```python
from build123d import *

# Parameters (mm, degrees)
SKETCH1_W           = 200
SKETCH1_H           = 100
BOSS_EXTRUDE1_DEPTH = 5
SKETCH2_W           = 50
SKETCH2_H           = 54
CUT_EXTRUDE1_DEPTH  = 6
SKETCH3_W           = 50
SKETCH3_H           = 4
BOSS_EXTRUDE2_DEPTH = 45
CUT_EXTRUDE3_DEPTH  = 4
SKETCH19_W          = 200
SKETCH19_H          = 5
BOSS_EXTRUDE3_DEPTH = 25
SKETCH20_W          = 200
SKETCH20_H          = 5
BOSS_EXTRUDE4_DEPTH = 25
SKETCH21_W          = 150
SKETCH21_H          = 5
BOSS_EXTRUDE5_DEPTH = 25
SKETCH22_OUTSIDE_W  = 282
SKETCH22_OUTSIDE_H  = 207
SKETCH22_OUTSIDE_R  = 75
CUT_EXTRUDE6_DEPTH  = 51
SKETCH26_R          = 2
CUT_EXTRUDE7_DEPTH  = 51
CUT_EXTRUDE8_REACH  = 52
SKETCH28_R          = 4.2
CUT_EXTRUDE10_DEPTH = 4


with BuildPart() as part:
    # Sketch1 → Boss-Extrude1 (new body)
    with BuildSketch(Plane(origin=(0, 0, 0), x_dir=(1, 0, 0), z_dir=(0, 1, 0))):
        Rectangle(SKETCH1_W, SKETCH1_H)
    extrude(amount=BOSS_EXTRUDE1_DEPTH)

    # Sketch2 → Cut-Extrude1 (cut, through all)
    with BuildSketch(Plane(origin=(0, 5, 0), x_dir=(1, 0, 0), z_dir=(0, 1, 0))):
        with Locations((30, 0)):
            Rectangle(SKETCH2_W, SKETCH2_H)
    extrude(amount=-CUT_EXTRUDE1_DEPTH, mode=Mode.SUBTRACT)

    # Sketch3 → Boss-Extrude2 (add)
    with BuildSketch(Plane.XZ):
        with Locations((30, -29)):
            Rectangle(SKETCH3_W, SKETCH3_H)
    extrude(amount=BOSS_EXTRUDE2_DEPTH)

    # Sketch4 → Cut-Extrude3 (cut)
    with BuildSketch(Plane.XY.offset(-27)):
        with BuildLine():
            ThreePointArc((14, 3.960327286), (11.85, 6.110327286), (9.7, 3.960327286))
            Line((9.7, 3.960327286), (9.7, -6.197738793))
            Line((9.7, -6.197738793), (14, -6.197264156))
            Line((14, -6.197264156), (14, 3.960327286))
        make_face()
        with BuildLine():
            Line((41.7, 3.960327286), (41.7, -31.94922721))
            ThreePointArc((41.7, -31.94922721), (43.85, -34.09922721), (46, -31.94922721))
            Line((46, -31.94922721), (46, 3.960327286))
            ThreePointArc((46, 3.960327286), (43.85, 6.110327286), (41.7, 3.960327286))
        make_face()
    extrude(amount=-CUT_EXTRUDE3_DEPTH, mode=Mode.SUBTRACT)

    # Sketch19 → Boss-Extrude3 (add)
    with BuildSketch(Plane(origin=(0, 0, -50), x_dir=(-1, 0, 0), z_dir=(0, 0, -1))):
        with Locations((0, 2.5)):
            Rectangle(SKETCH19_W, SKETCH19_H)
    extrude(amount=BOSS_EXTRUDE3_DEPTH)

    # Sketch20 → Boss-Extrude4 (add)
    with BuildSketch(Plane.XY.offset(50)):
        with Locations((0, 2.5)):
            Rectangle(SKETCH20_W, SKETCH20_H)
    extrude(amount=BOSS_EXTRUDE4_DEPTH)

    # Sketch21 → Boss-Extrude5 (add)
    with BuildSketch(Plane(origin=(100, 0, 0), x_dir=(0, 0, -1), z_dir=(1, 0, 0))):
        with Locations((0, 2.5)):
            Rectangle(SKETCH21_W, SKETCH21_H)
    extrude(amount=BOSS_EXTRUDE5_DEPTH)

    # Sketch22 outside → Cut-Extrude6 (cut, through all)
    with BuildSketch(Plane(origin=(0, 5, 0), x_dir=(1, 0, 0), z_dir=(0, 1, 0))):
        with Locations((12.5, 0)):
            Rectangle(SKETCH22_OUTSIDE_W, SKETCH22_OUTSIDE_H)
        with Locations((30, 0)):
            Circle(SKETCH22_OUTSIDE_R, mode=Mode.SUBTRACT)
    extrude(amount=-CUT_EXTRUDE6_DEPTH, mode=Mode.SUBTRACT)

    # Sketch26 → Cut-Extrude7 (cut, through all)
    with BuildSketch(Plane(origin=(0, 5, 0), x_dir=(1, 0, 0), z_dir=(0, 1, 0))):
        with Locations((30, -70)):
            Circle(SKETCH26_R)
        with Locations((-30.621778265, -35)):
            Circle(SKETCH26_R)
        with Locations((-30.621778265, 35)):
            Circle(SKETCH26_R)
        with Locations((30, 70)):
            Circle(SKETCH26_R)
        with Locations((90.621778265, 35)):
            Circle(SKETCH26_R)
        with Locations((90.621778265, -35)):
            Circle(SKETCH26_R)
    extrude(amount=-CUT_EXTRUDE7_DEPTH, mode=Mode.SUBTRACT)

    # Sketch28 → Cut-Extrude8 (cut, up to next)
    with BuildSketch(Plane(origin=(0, 5, 0), x_dir=(1, 0, 0), z_dir=(0, 1, 0)), mode=Mode.PRIVATE) as cut_extrude8_sk1:
        with Locations((-8.5, -3.95)):
            Circle(SKETCH28_R)
    cut_extrude8_tool1 = extrude(cut_extrude8_sk1.sketch, amount=-CUT_EXTRUDE8_REACH, mode=Mode.PRIVATE) & part.part
    add(cut_extrude8_tool1.solids().sort_by_distance((-8.5, 5, 3.95))[0], mode=Mode.SUBTRACT)
    # Sketch28 → Cut-Extrude8 (cut, up to next)
    with BuildSketch(Plane(origin=(0, 5, 0), x_dir=(1, 0, 0), z_dir=(0, 1, 0)), mode=Mode.PRIVATE) as cut_extrude8_sk2:
        with Locations((68.5, -3.95)):
            Circle(SKETCH28_R)
    cut_extrude8_tool2 = extrude(cut_extrude8_sk2.sketch, amount=-CUT_EXTRUDE8_REACH, mode=Mode.PRIVATE) & part.part
    add(cut_extrude8_tool2.solids().sort_by_distance((68.5, 5, 3.95))[0], mode=Mode.SUBTRACT)

    # Sketch30 → Cut-Extrude10 (cut)
    with BuildSketch(Plane.XY.offset(-27)):
        with BuildLine():
            Line((14, -6.197264156), (14, -40.571371384))
            ThreePointArc((14, -40.571371384), (11.85, -42.721371384), (9.7, -40.571371384))
            Line((9.7, -40.571371384), (9.7, -6.197738793))
            Line((9.7, -6.197738793), (14, -6.197264156))
        make_face()
        with BuildLine():
            Line((41.7, -31.94922721), (41.7, -36.94922721))
            ThreePointArc((41.7, -36.94922721), (43.85, -39.09922721), (46, -36.94922721))
            Line((46, -36.94922721), (46, -31.94922721))
            Line((46, -31.94922721), (41.7, -31.94922721))
        make_face()
    extrude(amount=-CUT_EXTRUDE10_DEPTH, mode=Mode.SUBTRACT)


solid = part.part
```
Read the model definition and answer for the solid it produces. Units are mm, in the model's axes. A direction names the side the tool comes from. Round coordinates to 2 decimals unless told otherwise and drop trailing zeros. Loops run counter-clockwise (first coordinate to the right, second up) from the corner with the lowest first, then second, coordinate; pieces in that order, holes last. Notation, with made-up numbers: (-28.5, 58.5) -> (29.5, 58.5) arc R25 ccw to (29.5, 73.5) -> close; hole circle Ø6 at (6.5, 21). An arc over 180 degrees is marked (long way). One line per item, written item: value.
1) A cutting plane is placed at A-A (y = -14.5). Determine the outline of the cut face in (x, z).
Answer list:
outline: (5, -31) -> (9.7, -31) -> (9.7, -27) -> (5, -27) -> close; (14, -31) -> (41.7, -31) -> (41.7, -27) -> (14, -27) -> close; (46, -31) -> (55, -31) -> (55, -27) -> (46, -27) -> close
2) A cutting plane is placed at D-D (x = -8.5). Determine the outline of the cut face in (y, z), and give its area (3 significant figures).
Answer list:
outline: (0, -64.36) -> (5, -64.36) -> (5, -0.25) -> (0, -0.25) -> close; (0, 8.15) -> (5, 8.15) -> (5, 64.36) -> (0, 64.36) -> close
area: 602 mm²
3) Consider L1, parallel to Z at x = 30, y = 1; L2, parallel to Y at x = 51, z = -54; L3, parallel to X at y = 2.65, z = -35. Determine where each line is inside the solid, lowest interval first. Write a range as [from, to].
Answer list:
L1: z = [-75, -72], [-68, -27], [27, 68], [72, 75]
L2: y = [0, 5]
L3: x = [-36.33, -32.62], [-28.62, 88.62], [92.62, 96.33]
4) The mould has two halves that part along Y. Classify faces 1 (the face through (41.7, -16, -29)), 2 (the face through (62, 5, 1)), 3 (the face through (-9.047, 2.535, -0.214)), 4 (the face through (30, -45, -29)): pulls with the +Y half, pulls with the -Y half, needs draft (parallel to the pull), parting line crosses it, or undercut.
Answer list:
face 1: undercut
face 2: pulls with the +Y half
face 3: needs draft
face 4: pulls with the -Y half
5) For faces 5 (the face through (30, -22, -31)), 6 (the face through (43.8, -39.1, -29)), 7 (the face through (5, 3, 0)), determine the directions among +Z, -Z, +X, -X, +Y, -Y from which every point of the face is accessible in a straight line to the end or side of a thin tool.
Answer list:
face 5: -Z, +X, -X, -Y
face 6: +Z, -Z
face 7: +Y, -Y
6) Flat-ended cylindrical pins translate along their axes: P1, Ø3, axis at y = -33, z = -29, coming from the -X side; P2, Ø6.5, axis at x = -30.62, z = 35, coming from the -Y side; P3, Ø1.2, axis at y = -19.5, z = -30, coming from the +X side. Find the tip coordinate at first contact, or state that the pin passes through.
Answer list:
P1: stops at x = 5
P2: stops at y = 0
P3: stops at x = 55
7) A cutting plane is placed at B-B (x = 30). Determine the outline of the cut face in (y, z), and give its area (3 significant figures).
Answer list:
outline: (-45, -31) -> (0, -31) -> (0, -68) -> (5, -68) -> (5, -27) -> (-45, -27) -> close; (0, -75) -> (5, -75) -> (5, -72) -> (0, -72) -> close; (0, 27) -> (5, 27) -> (5, 68) -> (0, 68) -> close; (0, 72) -> (5, 72) -> (5, 75) -> (0, 75) -> close
area: 620 mm²
8) A cutting plane is placed at C-C (z = -35). Determine the outline of the cut face in (x, y), and give its area (3 significant figures).
Answer list:
outline: (-36.33, 0) -> (-32.62, 0) -> (-32.62, 5) -> (-36.33, 5) -> close; (-28.62, 0) -> (88.62, 0) -> (88.62, 5) -> (-28.62, 5) -> close; (92.62, 0) -> (96.33, 0) -> (96.33, 5) -> (92.62, 5) -> close
area: 623 mm²
